```python
from build123d import *

# Parameters (mm, degrees)
SKETCH1_W                                     = 680
SKETCH1_H                                     = 150
VERTICAL_PORTION_DEPTH                        = 10
SHAFT_ADAPTER_RIGHT_DEPTH                     = 25
SHAFT_ADAPTER_FILLETS_R                       = 5
SKETCH5_W                                     = 100
SKETCH5_H                                     = 5
LIMIT_TAB_PREVENTS_GATE_FROM_GETTING_PU_DEPTH = 10
LIMIT_TAB_FILLETS_R                           = 5


with BuildPart() as part:
    # Sketch1 → Vertical portion (new body)
    with BuildSketch(Plane.XY):
        Rectangle(SKETCH1_W, SKETCH1_H)
    extrude(amount=VERTICAL_PORTION_DEPTH)

    # Sketch4 → Shaft adapter right (add)
    with BuildSketch(Plane(origin=(325, 0, 0), x_dir=(0, 0, -1), z_dir=(1, 0, 0))):
        with BuildLine():
            Line((-10, 45), (-30, 52.5))
            Line((-30, 52.5), (-30, 60))
            Line((-30, 60), (-25, 60))
            ThreePointArc((-25, 60), (-20, 55), (-15, 60))
            Line((-15, 60), (-10, 60))
            Line((-10, 60), (-10, 55))
            Line((-10, 55), (-10, 45))
        make_face()
    shaft_adapter_right = extrude(amount=-SHAFT_ADAPTER_RIGHT_DEPTH)

    # Shaft adapter left: Shaft adapter right across plane
    add(shaft_adapter_right.mirror(Plane(origin=(0, 0, 0), x_dir=(0, 0, 1), z_dir=(1, 0, 0))))

    # Shaft adapter fillets
    shaft_adapter_fillets_edges = [part.edges().sort_by_distance(p)[0] for p in [
        (-312.5, 52.5, 30),
        (312.5, 52.5, 30),
        (300, 52.5, 10),
        (-300, 52.5, 10),
        (-312.5, 45, 10),
        (312.5, 45, 10),
        (312.5, 60, 10),
        (-312.5, 60, 10),
    ]]
    fillet(shaft_adapter_fillets_edges, radius=SHAFT_ADAPTER_FILLETS_R - 0.0001)  # a hair under: the kernel refuses the full size

    # Sketch5 → Limit tab (prevents gate from getting pushed out of slot) (add)
    with BuildSketch(Plane(origin=(0, 0, 0), x_dir=(-1, 0, 0), z_dir=(0, 0, -1))):
        with Locations((-100, -72.5)):
            Rectangle(SKETCH5_W, SKETCH5_H)
        with Locations((100, -72.5)):
            Rectangle(SKETCH5_W, SKETCH5_H)
    extrude(amount=LIMIT_TAB_PREVENTS_GATE_FROM_GETTING_PU_DEPTH)

    # Limit tab fillets
    limit_tab_fillets_edges = [part.edges().sort_by_distance(p)[0] for p in [
        (150, -72.5, 0),
        (50, -72.5, 0),
        (100, -70, 0),
        (-150, -72.5, 0),
        (-100, -70, 0),
        (-50, -72.5, 0),
    ]]
    fillet(limit_tab_fillets_edges, radius=LIMIT_TAB_FILLETS_R)


solid = part.part
```
Check sheet for the modelled part. Datum: model origin and axes. Units: mm. A direction names the side the tool comes from. Coordinates: 2 decimals unless noted, no trailing zeros. Loops run counter-clockwise (first coordinate to the right, second up) from the corner with the lowest first, then second, coordinate; pieces in that order, holes last. Notation, with made-up numbers: M 79.5,46 L 116.5,46 A25 ccw 116.5,78 Z; hole C 87,-19.75 d8. An arc over 180 degrees is marked long. Answer as a JSON object with one key per item and string values.
1. Sectioned sample at B-B on y = -18. Record the cut outline in (x, z).
Outcome:
{"outline": "M -340,0 L 340,0 L 340,10 L -340,10 Z"}
2. Sectioned sample at A-A on x = 62. Record the cut outline in (y, z).
Outcome:
{"outline": "M -75,-10 L -70,-10 L -70,-5 A5 cw -65,0 L 75,0 L 75,10 L -75,10 Z"}
3. Depth check by flat-ended pin: P1, Ø1.5, axis at x = 7.5, y = 20, coming from the -Z side; P2, Ø2.5, axis at x = -99, z = -8.5, coming from the +Y side; P3, Ø10, axis at y = 52.5, z = 22.5, coming from the +X side; P4, Ø16, axis at y = 52.5, z = 16, coming from the -X side. Enter the tip coordinate at first touch or a pass-through.
Outcome:
{"P1": "z = 0", "P2": "y = -70", "P3": "x = 325", "P4": "x = -340"}
4. Sectioned sample at C-C on x = -200. Record the cut outline in (y, z), and give its area (3 significant figures).
Outcome:
{"outline": "M -75,0 L 75,0 L 75,10 L -75,10 Z", "area": "1,500 mm²"}
5. Release check for a two-part mould opening along X. For faces 1 (the flat face through (325, 53, 18)), 2 (the flat face through (312.518, 48.715, 19.905)), 3 (the flat face through (-300, 54, 22)) record: pulls with the +X half, pulls with the -X half, needs draft (parallel to the pull), parting line crosses it, or undercut.
Outcome:
{"face 1": "pulls with the +X half", "face 2": "needs draft", "face 3": "undercut"}
6. Scan line: L1, parallel to Z at x = -33, y = -13.5. Record every from-to range of solid material in increasing order. Write a range as from..to.
Outcome:
{"L1": "0..10"}
7. Access from +Z, -Z, +X, -X, +Y, -Y to the whole of each face (thin tool, end or side, straight path). Record for faces 4 (the flat face through (300, 54, 22)), 5 (the flat face through (-5, -75, 2)), 6 (the flat face through (-325, 53, 18)).
Outcome:
{"face 4": "+Z, +Y, -Y", "face 5": "+Z, -Z, +X, -X, -Y", "face 6": "+Z, -X, +Y, -Y"}
